Here's how the part is built. I have some questions about the finished solid (model axes, mm). Face numbers are marked on the shaded views. A direction names the side the tool comes from. Round coordinates to 2 decimals unless told otherwise and drop trailing zeros. Loops run counter-clockwise (first coordinate to the right, second up) from the corner with the lowest first, then second, coordinate; pieces in that order, holes last. Notation, with made-up numbers: M 64,71 L 85,71 A18 ccw 85,88 Z; hole C 48.25,71 d7. An arc over 180 degrees is marked long. Use a Markdown table: item, result.
```python
from build123d import *

# Parameters (mm, degrees)
SKIZZE1_W                       = 20
SKIZZE1_H                       = 20
AUFSATZ_LINEAR_AUSTRAGEN1_DEPTH = 2
AUFSATZ_LINEAR_AUSTRAGEN3_DEPTH = 5
VERRUNDUNG1_R                   = 3
VERRUNDUNG1_OF_SPIEGELN1_R      = 3
AUFSATZ_LINEAR_AUSTRAGEN4_REACH = 22.848
SKIZZE3_W                       = 37.447689889
SKIZZE3_H                       = 20
SKIZZE4_R                       = 1.75
SCHNITT_LINEAR_AUSTRAGEN1_DEPTH = 21
SKIZZE4_3_R                     = 2.9
SKIZZE4_3_R_2                   = 1.75
SCHNITT_LINEAR_AUSTRAGEN2_DEPTH = 16
AUFSATZ_LINEAR_AUSTRAGEN5_REACH = 27.254
SKIZZE5_W                       = 2.691263413
SKIZZE5_H                       = 6


with BuildPart() as part:
    # Skizze1 → Aufsatz-Linear austragen1 (new body)
    with BuildSketch(Plane.XY):
        with Locations((10, 10)):
            Rectangle(SKIZZE1_W, SKIZZE1_H)
    aufsatz_linear_austragen1 = extrude(amount=AUFSATZ_LINEAR_AUSTRAGEN1_DEPTH)

    # Skizze2 → Aufsatz-Linear austragen3 (add)
    with BuildSketch(Plane.XY.offset(2)):
        with BuildLine():
            Line((13, 18.1), (13, 20))
            Line((13, 20), (7, 20))
            Line((7, 20), (7, 18.1))
            Line((7, 18.1), (5.883086579, 18.1))
            ThreePointArc((5.883086579, 18.1), (5.147285539, 17.57883746), (5.394745881, 16.711786745))
            Line((5.394745881, 16.711786745), (7.506532626, 14.6))
            Line((7.506532626, 14.6), (9.080240322, 14.6))
            Line((9.080240322, 14.6), (10.919759678, 14.6))
            Line((10.919759678, 14.6), (12.493467374, 14.6))
            Line((12.493467374, 14.6), (14.605254119, 16.711786745))
            ThreePointArc((14.605254119, 16.711786745), (14.852714461, 17.57883746), (14.116913421, 18.1))
            Line((14.116913421, 18.1), (13, 18.1))
        make_face()
        with BuildLine():
            Line((1.9, 13), (0, 13))
            Line((0, 13), (0, 7))
            Line((0, 7), (1.9, 7))
            Line((1.9, 7), (1.9, 5.883086579))
            ThreePointArc((1.9, 5.883086579), (2.42116254, 5.147285539), (3.288213255, 5.394745881))
            Line((3.288213255, 5.394745881), (4.739281749, 7.20200687))
            ThreePointArc((4.739281749, 7.20200687), (5.230003997, 8.08471163), (5.4, 9.080240322))
            Line((5.4, 9.080240322), (5.4, 10.919759678))
            ThreePointArc((5.4, 10.919759678), (5.230003997, 11.91528837), (4.739281749, 12.79799313))
            Line((4.739281749, 12.79799313), (3.288213255, 14.605254119))
            ThreePointArc((3.288213255, 14.605254119), (2.42116254, 14.852714461), (1.9, 14.116913421))
            Line((1.9, 14.116913421), (1.9, 13))
        make_face()
        with BuildLine():
            Line((7, 0), (13, 0))
            Line((13, 0), (13, 1.9))
            Line((13, 1.9), (14.116913421, 1.9))
            ThreePointArc((14.116913421, 1.9), (14.852714461, 2.42116254), (14.605254119, 3.288213255))
            Line((14.605254119, 3.288213255), (12.315477065, 5.577990309))
            ThreePointArc((12.315477065, 5.577990309), (11.607035992, 5.571977263), (10.919759678, 5.4))
            Line((10.919759678, 5.4), (9.080240322, 5.4))
            ThreePointArc((9.080240322, 5.4), (8.392964008, 5.571977263), (7.684522935, 5.577990309))
            Line((7.684522935, 5.577990309), (5.394745881, 3.288213255))
            ThreePointArc((5.394745881, 3.288213255), (5.147285539, 2.42116254), (5.883086579, 1.9))
            Line((5.883086579, 1.9), (7, 1.9))
            Line((7, 1.9), (7, 0))
        make_face()
        with BuildLine():
            Line((20, 7), (20, 13))
            Line((20, 13), (18.1, 13))
            Line((18.1, 13), (18.1, 14.116913421))
            ThreePointArc((18.1, 14.116913421), (17.57883746, 14.852714461), (16.711786745, 14.605254119))
            Line((16.711786745, 14.605254119), (15.260718251, 12.79799313))
            ThreePointArc((15.260718251, 12.79799313), (14.769996003, 11.91528837), (14.6, 10.919759678))
            Line((14.6, 10.919759678), (14.6, 9.080240322))
            ThreePointArc((14.6, 9.080240322), (14.769996003, 8.08471163), (15.260718251, 7.20200687))
            Line((15.260718251, 7.20200687), (16.711786745, 5.394745881))
            ThreePointArc((16.711786745, 5.394745881), (17.57883746, 5.147285539), (18.1, 5.883086579))
            Line((18.1, 5.883086579), (18.1, 7))
            Line((18.1, 7), (20, 7))
        make_face()
    aufsatz_linear_austragen3 = extrude(amount=AUFSATZ_LINEAR_AUSTRAGEN3_DEPTH)

    # Verrundung1
    verrundung1_edges = [part.edges().sort_by_distance(p)[0] for p in [
        (7.506532626, 14.6, 4.5),
        (12.493467374, 14.6, 4.5),
    ]]
    fillet(verrundung1_edges, radius=VERRUNDUNG1_R)

    # Spiegeln1: Aufsatz-Linear austragen1, Aufsatz-Linear austragen3 across plane
    add(aufsatz_linear_austragen1.mirror(Plane(origin=(0.518393786, 0, 0.144857975), x_dir=(-0.269126341, 0, 0.963104881), z_dir=(-0.963104881, 0, -0.269126341))))
    add(aufsatz_linear_austragen3.mirror(Plane(origin=(0.518393786, 0, 0.144857975), x_dir=(-0.269126341, 0, 0.963104881), z_dir=(-0.963104881, 0, -0.269126341))))

    # Verrundung1 of Spiegeln1
    verrundung1_of_spiegeln1_edges = [part.edges().sort_by_distance(p)[0] for p in [
        (-7.715135975, 14.6, 0.246515195),
        (-11.979673452, 14.6, -2.338680788),
    ]]
    fillet(verrundung1_of_spiegeln1_edges, radius=VERRUNDUNG1_OF_SPIEGELN1_R)

    # Skizze3 → Aufsatz-Linear austragen4 (add, up to next)
    with BuildSketch(Plane(origin=(2.36988033, 0, -8.480936141), x_dir=(-0.963104881, 0, -0.269126341), z_dir=(0.269126341, 0, -0.963104881)), mode=Mode.PRIVATE) as aufsatz_linear_austragen4_sk1:
        with Locations((-0.538252683, 10)):
            Rectangle(SKIZZE3_W, SKIZZE3_H)
    aufsatz_linear_austragen4_tool1 = extrude(aufsatz_linear_austragen4_sk1.sketch, amount=-AUFSATZ_LINEAR_AUSTRAGEN4_REACH, mode=Mode.PRIVATE) - part.part
    add(aufsatz_linear_austragen4_tool1.solids().sort_by_distance((2.888274, 10, -8.336078))[0])

    # Skizze4 → Schnitt-Linear austragen1 (cut, through all)
    with BuildSketch(Plane.XZ):
        with Locations((1.495339923, -3.351275437)):
            Circle(SKIZZE4_R)
    extrude(amount=-SCHNITT_LINEAR_AUSTRAGEN1_DEPTH, mode=Mode.SUBTRACT)

    # Skizze4<3> → Schnitt-Linear austragen2 (cut)
    with BuildSketch(Plane.XZ):
        with Locations((1.495339923, -3.351275437)):
            Circle(SKIZZE4_3_R)
        with Locations((1.495339923, -3.351275437)):
            Circle(SKIZZE4_3_R_2, mode=Mode.SUBTRACT)
    extrude(amount=-SCHNITT_LINEAR_AUSTRAGEN2_DEPTH, mode=Mode.SUBTRACT)

    # Skizze5 → Aufsatz-Linear austragen5 (add, up to next)
    with BuildSketch(Plane(origin=(-1.814378251, 0, 6.492997087), x_dir=(0.963104881, 0, 0.269126341), z_dir=(-0.269126341, 0, 0.963104881)), mode=Mode.PRIVATE) as aufsatz_linear_austragen5_sk1:
        with Locations((0.538252683, 10)):
            Rectangle(SKIZZE5_W, SKIZZE5_H)
    aufsatz_linear_austragen5_tool1 = extrude(aufsatz_linear_austragen5_sk1.sketch, amount=-AUFSATZ_LINEAR_AUSTRAGEN5_REACH, mode=Mode.PRIVATE) - part.part
    add(aufsatz_linear_austragen5_tool1.solids().sort_by_distance((-1.295984, 10, 6.637855))[0])


solid = part.part
```
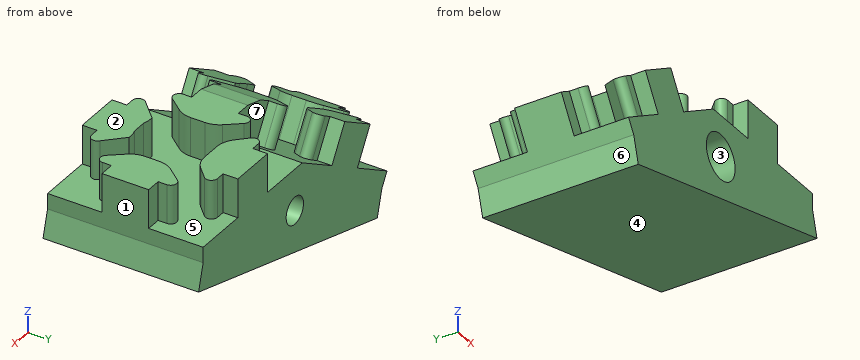
Q1. Will these pins go through, and if not, where does the flat tip stop? P1, Ø1, axis at x = 11.5, y = 14, coming from the -Z side; P2, Ø1.3, axis at x = -17.5, z = -4.5, coming from the +Y side; P3, Ø1, axis at y = 1, z = 4.5, coming from the +X side.
Return value:
| item | result |
|---|---|
| P1 | stops at z = -6.07 |
| P2 | stops at y = 14.81 |
| P3 | stops at x = 13 |
Q2. Imagine slicing it at B-B, the plane x = -1. Please give me the cut outline in (y, z), then the cut area to 3 significant figures.
Return value:
| item | result |
|---|---|
| outline | M 0,-9.42 L 20,-9.42 L 20,1.39 L 13,1.39 L 13,6.72 L 7,6.72 L 7,1.39 L 0,1.39 L 0,-1.87 L 16,-1.87 L 16,-4.83 L 0,-4.83 Z |
| area | 201 mm^2 |
Q3. Imagine slicing it at C-C, the plane z = -11. Please give me the cut outline in (x, y).
Return value:
| item | result |
|---|---|
| outline | M -15.81,0 L -6.64,0 L -6.64,20 L -15.81,20 Z |
Q4. Imagine slicing it at A-A, the plane y = 13.5. Please give me the cut outline in (x, z).
Return value:
| item | result |
|---|---|
| outline | M -18.07,-3.11 L -15.48,-7.38 L -17.1,-8.37 L -16.07,-10.08 L -15.14,-13.38 L 20.92,-3.3 L 20,0 L 20,2 L 18.1,2 L 18.1,7 L 15.82,7 L 15.82,2 L 4.18,2 L 4.18,7 L 1.9,7 L 1.9,2 L 0,2 L -1.62,1.02 L -4.22,5.29 L -6.16,4.11 L -3.57,-0.16 L -13.53,-6.2 L -16.12,-1.93 Z; hole C 1.5,-3.35 d5.8 |
Q5. I need wall thicknesses on line 1 (Y direction, x = -7, z = -1.5); line 2 (Y direction, x = 14, z = 5.75); line 3 (X direction, y = 18, z = -3). Which ranges of each line are inside material? Lowest first, please. Write a range as from..to.
Return value:
| item | result |
|---|---|
| line 1 | y = 0..5.59, 14.75..20 |
| line 2 | y = 1.9..3.89, 16.11..18.1 |
| line 3 | x = -13.92..-0.22, 3.21..20.84 |
Q6. For the marked faces 5, 6 and 7, which set-ups out of +Z, -Z, +X, -X, +Y, -Y let a thin tool reach every point of the face, with its end or its side?
Return value:
| item | result |
|---|---|
| face 5 | +Z |
| face 6 | -Z, -X, +Y, -Y |
| face 7 | +Z, +Y |
Q7. We'd pull the mould along Z, two halves only. Please class the marked faces 1, 2, 3 and 4: pulls with the +Z half, pulls with the -Z half, needs draft (parallel to the pull), parting line crosses it, or undercut.
Return value:
| item | result |
|---|---|
| face 1 | needs draft |
| face 2 | pulls with the +Z half |
| face 3 | undercut |
| face 4 | pulls with the -Z half |
